from build123d import *

# Parameters (mm, degrees)
CROQUIS1_W              = 100
CROQUIS1_H              = 50
SALIENTE_EXTRUIR1_DEPTH = 30
CROQUIS2_W              = 70
CROQUIS2_H              = 25
SALIENTE_EXTRUIR2_DEPTH = 40
CROQUIS3_W              = 50
CROQUIS3_H              = 25
SALIENTE_EXTRUIR3_DEPTH = 30
CROQUIS4_R              = 20
CORTAR_EXTRUIR1_DEPTH   = 83.006097334
CHAFL_N1_SIZE           = 2
CROQUIS5_W              = 60
CROQUIS5_H              = 5
CORTAR_EXTRUIR2_DEPTH   = 90.582364336
REDONDEO1_R             = 10
REDONDEO2_R             = 5
CROQUIS6_R              = 5
CORTAR_EXTRUIR3_DEPTH   = 69.738635424
SALIENTE_EXTRUIR4_DEPTH = 1


with BuildPart() as part:
    # Croquis1 → Saliente-Extruir1 (new body)
    with BuildSketch(Plane.XY):
        Rectangle(CROQUIS1_W, CROQUIS1_H)
    extrude(amount=SALIENTE_EXTRUIR1_DEPTH)

    # Croquis2 → Saliente-Extruir2 (add)
    with BuildSketch(Plane.XY.offset(30)):
        with Locations((0, -12.5)):
            Rectangle(CROQUIS2_W, CROQUIS2_H)
    extrude(amount=SALIENTE_EXTRUIR2_DEPTH)

    # Croquis3 → Saliente-Extruir3 (add)
    with BuildSketch(Plane.XY.offset(30)):
        with Locations((0, 12.5)):
            Rectangle(CROQUIS3_W, CROQUIS3_H)
    extrude(amount=SALIENTE_EXTRUIR3_DEPTH)

    # Croquis4 → Cortar-Extruir1 (cut, through all)
    with BuildSketch(Plane.XY.offset(60)):
        with Locations((0, 25)):
            Circle(CROQUIS4_R)
    extrude(amount=-CORTAR_EXTRUIR1_DEPTH, mode=Mode.SUBTRACT)

    # Chaflán1
    chafl_n1_edges = [part.edges().sort_by_distance(p)[0] for p in [
        (0, 5, 60),
    ]]
    chamfer(chafl_n1_edges, length=CHAFL_N1_SIZE)

    # Croquis5 → Cortar-Extruir2 (cut, through all)
    with BuildSketch(Plane.XY.offset(70)):
        with Locations((0, -22.5)):
            Rectangle(CROQUIS5_W, CROQUIS5_H)
    extrude(amount=-CORTAR_EXTRUIR2_DEPTH, mode=Mode.SUBTRACT)

    # Redondeo1
    redondeo1_edges = [part.edges().sort_by_distance(p)[0] for p in [
        (-50, 25, 15),
        (50, 25, 15),
    ]]
    fillet(redondeo1_edges, radius=REDONDEO1_R)

    # Redondeo2
    redondeo2_edges = [part.edges().sort_by_distance(p)[0] for p in [
        (-35, 0, 50),
        (35, 0, 50),
        (-25, 12.5, 30),
        (25, 12.5, 30),
    ]]
    fillet(redondeo2_edges, radius=REDONDEO2_R - 0.0001)  # a hair under: the kernel refuses the full size

    # Croquis6 → Cortar-Extruir3 (cut, through all)
    with BuildSketch(Plane.XY.offset(30)):
        with Locations((-40, 15)):
            Circle(CROQUIS6_R)
        with Locations((40, 15)):
            Circle(CROQUIS6_R)
    extrude(amount=-CORTAR_EXTRUIR3_DEPTH, mode=Mode.SUBTRACT)

    # Croquis9 → Saliente-Extruir4 (add)
    with BuildSketch(Plane.XY.offset(30)):
        Polygon((-40, 21.494353202), (-44.592201188, 19.592201188), (-46.494353202, 15), (-44.592201188, 10.407798812), (-40, 8.505646798), (-35.407798812, 10.407798812), (-33.505646798, 15), (-35.407798812, 19.592201188), align=None)
        Polygon((40, 21.494353202), (35.407798812, 19.592201188), (33.505646798, 15), (35.407798812, 10.407798812), (40, 8.505646798), (44.592201188, 10.407798812), (46.494353202, 15), (44.592201188, 19.592201188), align=None)
    extrude(amount=SALIENTE_EXTRUIR4_DEPTH)


solid = part.part
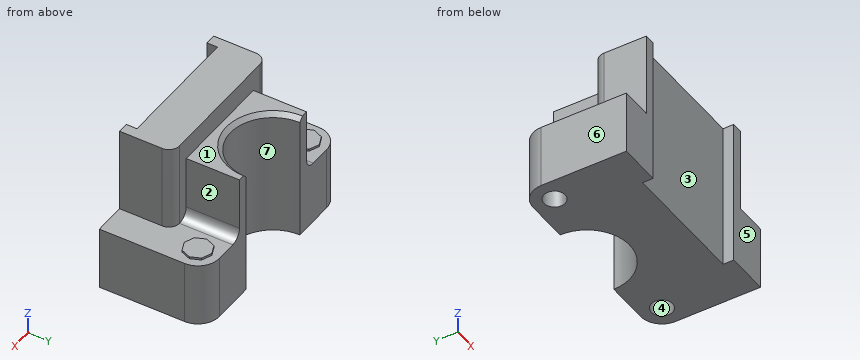
Design review of the part built by this model. Coordinates are the model's own, in mm. Face numbers are marked on the shaded views. A direction names the side the tool comes from. Round coordinates to 2 decimals unless told otherwise and drop trailing zeros. Loops run counter-clockwise (first coordinate to the right, second up) from the corner with the lowest first, then second, coordinate; pieces in that order, holes last. Notation, with made-up numbers: (-12, 6.25) - (27, 6.25) arc R32 ccw to (27, 35.25) - close; hole circle Ø10 at (68, 43.25). An arc over 180 degrees is marked (long way). One line per item, written item: value. Start each with the question number.
1) Consider section B-B on z = 5. Give the boundary of the cut face in (x, y), then the cut area to 3 significant figures.
2) Consider section C-C on y = 1.5. Give the boundary of the cut face in (x, z), then the cut area to 3 significant figures.
3) Draft analysis for pull direction X (two halves, no side actions). For the marked faces 5, 6 and 7, state which applies: +X half, -X half, draft (parallel to the pull), parting line (faces both ways), or undercut.
4) For the marked faces 1, 2, 3 and 4, list the 3-axis set-ups (+Z, -Z, +X, -X, +Y, -Y) from which the entire face can be reached by the end or side of a thin tool; tool diameter is ignored.
5) Consider section D-D on z = 53. Give the boundary of the cut face in (x, y).
6) Insertion check: pin 1 Ø20 at (y, z) = (8.5, 49) entering from -X; pin 2 Ø6 at (x, y) = (-41.5, 3.5) entering from +Z; pin 3 Ø5 at (x, y) = (39, 14) entering from -Z. Each pin has a flat end and moves straight along its axis. Give the tip position at first contact, or say it passes through.
7) To check wall thickness, follow L1, parallel to Y at x = -40, z = 18.25; L2, parallel to X at y = -21.5, z = 67; L3, parallel to Z at x = -9.5, y = 1. State the ranges of each line that lie inside material, in increasing order. Write a range as from..to.
8) Consider section A-A on x = 0. Give the boundary of the cut face in (y, z), then the cut area to 3 significant figures.
Reported:
1. outline: (-50, -25) - (-30, -25) - (-30, -20) - (30, -20) - (30, -25) - (50, -25) - (50, 15) arc R10 ccw to (40, 25) - (20, 25) arc R20 cw to (-20, 25) - (-40, 25) arc R10 ccw to (-50, 15) - close; hole circle Ø10 at (-40, 15); hole circle Ø10 at (40, 15)
1. area: 3,870 mm^2
2. outline: (-50, 0) - (50, 0) - (50, 30) - (30, 30) arc R5 cw to (25, 35) - (25, 60) - (-25, 60) - (-25, 35) arc R5 cw to (-30, 30) - (-50, 30) - close
2. area: 4,510 mm^2
3. face 5: draft
3. face 6: -X half
3. face 7: undercut
4. face 1: +Z, +X, -X, +Y
4. face 2: +Z, +X, +Y
4. face 3: +Z, -Z, -Y
4. face 4: -Z
5. outline: (-35, -25) - (-30, -25) - (-30, -20) - (30, -20) - (30, -25) - (35, -25) - (35, -5) arc R5 ccw to (30, 0) - (25, 0) - (25, 25) - (20, 25) arc R20 cw to (-20, 25) - (-25, 25) - (-25, 0) - (-30, 0) arc R5 ccw to (-35, -5) - close
6. pin 1: stops at x = -33.57
6. pin 2: stops at z = 30
6. pin 3: stops at z = 30
7. L1: y = -25..10, 20..25
7. L2: x = -35..-30, 30..35
7. L3: z = 0..60
8. outline: (-20, 0) - (5, 0) - (5, 58) - (3, 60) - (0, 60) - (0, 70) - (-20, 70) - close
8. area: 1,700 mm^2
